Build history of the part. All positions in model axes, mm. Face numbers are marked on the shaded views. A direction names the side the tool comes from. Give positions to 0.01 mm unless a question says otherwise; leave off trailing zeros. Order: outer loops, then holes, each group sorted by start corner. A loop starts at its lowest first (then second) coordinate and runs counter-clockwise, first axis right, second up. Notation, with made-up numbers: (50, -4.75) - (95, -4.75) arc R24 cw to (95, 33.25) - close; hole circle Ø11 at (41.5, 73.25). An arc over 180 degrees is marked (long way). One line per item, written item: value.
Autodesk Inventor part; units mm, degrees
ref_plane "YZ Plane" through (0, 0, 0) normal (1, 0, 0) x (0, 1, 0)
ref_plane "XZ Plane" through (0, 0, 0) normal (0, 1, 0) x (-1, 0, 0)
ref_plane "XY Plane" through (0, 0, 0) normal (0, 0, 1) x (1, 0, 0)
sketch "Sketch1" plane through (0, 0, 0) normal (0, 0, 1) x (1, 0, 0)
  line L0 (0, 0) -> (27, 0)
  line L1 (30, -3) -> (30, -30)
  arc A0 (30, -3) -> (27, 0) centre (27, -3) ccw
  point P0 (30, 0)
  dimension "d0" = 30
  dimension "d1" = 30
  dimension "d7" = 3
sketch "Sketch2" plane through (0, 0, 0) normal (1, 0, 0) x (0, 1, 0)
  line L0 (0, 0) -> (0, -10)
  line L1 (0, -10) -> (1, -10)
  line L2 (1, -10) -> (1, 0)
  line L3 (1, 0) -> (0, 0)
  dimension "d2" = 10
  dimension "d3" = 1
  dimension "d4" = 10
sweep "Sweep1" add profiles "Sketch2" path "Sketch1"
hole "Hole1" at (5, 1, -3.5) direction (0, -1, 0) diameter 4 end through all
hole "Hole2" at (22, 1, -6.5) direction (0, -1, 0) diameter 4 end through all
hole "Hole3" at (31, -8, -6.5) direction (-1, 0, 0) diameter 4 end through all
hole "Hole4" at (31, -25, -3.5) direction (-1, 0, 0) diameter 4 end through all
chamfer "Chamfer1" distance 0.25 angle 45 4 edges at (5, 0, -5.5) (22, 0, -8.5) (30, -8, -4.5) (30, -25, -1.5)
properties part number "30mmCornerBracket"
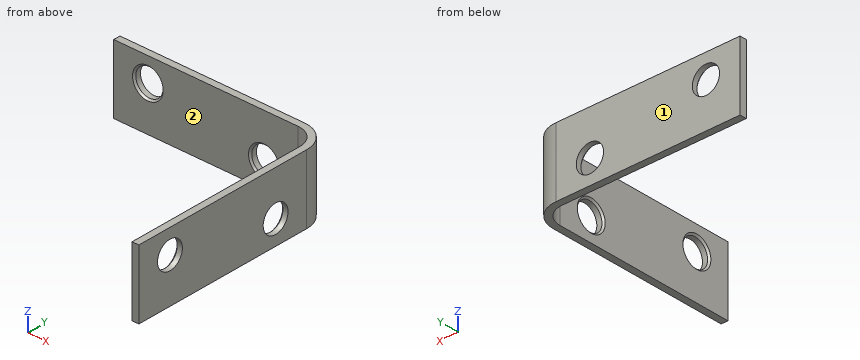
(1) Slice it at D-D, the plane y = -18. Give the cut face in (x, z), and give its area (3 significant figures).
Completed:
outline: (30, -10) - (31, -10) - (31, 0) - (30, 0) - close
area: 10.0 mm²
(2) Slice it at A-A, the plane x = 22. Give the cut face in (y, z).
Completed:
outline: (0, -10) - (1, -10) - (1, -8.5) - (0.25, -8.5) - (0, -8.75) - close; (0, -4.25) - (0.25, -4.5) - (1, -4.5) - (1, 0) - (0, 0) - close
(3) Pin check, flat tips, straight feed: P1, Ø5, axis at y = -5, z = -3, coming from the -X side; P2, Ø2, axis at x = 4, z = -9, coming from the -Y side. Stop position of each tip, or through.
Completed:
P1: x = 29.96
P2: y = 0
(4) Slice it at C-C, the plane z = -6.5. Give the cut face in (x, y), and give its area (3 significant figures).
Completed:
outline: (0, 0) - (19.75, 0) - (20, 0.25) - (20, 1) - (0, 1) - close; (24, 0.25) - (24.25, 0) - (27, 0) arc R3 cw to (30, -3) - (30, -5.75) - (30.25, -6) - (31, -6) - (31, -3) arc R4 ccw to (27, 1) - (24, 1) - close; (30, -30) - (31, -30) - (31, -10) - (30.25, -10) - (30, -10.25) - close
area: 51.4 mm²
(5) Slice it at B-B, the plane y = -25. Give the cut face in (x, z).
Completed:
outline: (30, -10) - (31, -10) - (31, -5.5) - (30.25, -5.5) - (30, -5.75) - close; (30, -1.25) - (30.25, -1.5) - (31, -1.5) - (31, 0) - (30, 0) - close
(6) 3-axis set-ups, long thin cutter, end or side, ignore diameter. For the marked faces 1 and 2: which of +Z, -Z, +X, -X, +Y, -Y reach the whole face in a straight line?
Completed:
face 1: +Z, -Z, +X, -X, +Y
face 2: +Z, -Z, -X, -Y
(7) Drill centre lines: line 1 (Z direction, x = 5, y = 0.45); line 2 (Z direction, x = 22, y = 0.8); line 3 (Y direction, x = 30.6, z = -3.5). Where is each one in solid material? Low to high.
Completed:
line 1: -10 to -5.5, -1.5 to 0
line 2: -10 to -8.5, -4.5 to 0
line 3: -30 to -27, -23 to -1.26
